Check sheet for the modelled part. Datum: model origin and axes. Units: mm. A direction names the side the tool comes from. Round coordinates to 2 decimals unless told otherwise and drop trailing zeros. Loops run counter-clockwise (first coordinate to the right, second up) from the corner with the lowest first, then second, coordinate; pieces in that order, holes last. Notation, with made-up numbers: (-36.75, -27.5) -> (7.25, -27.5) arc R22 cw to (7.25, -6.5) -> close; hole circle Ø8 at (85.25, 69). An arc over 180 degrees is marked (long way). One line per item, written item: value. Start each with the question number.
1. Cross-section at C-C on x = -41.5. Record the cut outline in (y, z).
2. Set-up check for faces 5 (the face through (-76, 2.845, 2)), 6 (the face through (76.353, 1.402, -1.021)): record each of +Z, -Z, +X, -X, +Y, -Y from which the full face is reachable in a straight line by a thin tool's end or side.
3. Cross-section at A-A on x = 0. Record the cut outline in (y, z).
4. Cross-section at B-B on z = 0. Record the cut outline in (x, y), then the cut area to 3 significant figures.
5. Material ranges on L1, parallel to X at y = 1.2, z = 0; L2, parallel to X at y = 4.2, z = 0; L3, parallel to Z at x = 51, y = 0.5, recorded low to high.
6. Go/stop test with flat-tipped pins: pin 1 (3.5 mm diameter, centred on x = -1.5, z = -75, fed in from +Y); pin 2 (11.5 mm diameter, centred on x = 74.75, z = 0, fed in from +Y); pin 3 (3 mm diameter, centred on y = 2.5, z = 62, fed in from -X); pin 4 (1 mm diameter, centred on y = 2, z = -14, fed in from -X). Record where each tip stops, or that it passes through.
7. Release check for a two-part mould opening along X. For faces 1 (the face through (32.42, 3.13, 62.33)), 2 (the face through (-1.368, 4.622, -71.452)), 3 (the face through (-6, 6.35, -71)), 4 (the face through (-10.317, 3.131, -78.574)) record: +X half, -X half, draft (parallel to the pull), parting line (faces both ways), or undercut.
8. Cross-section at D-D on z = 57. Record the cut outline in (x, y).
from build123d import *

# Parameters (mm, degrees)
SKETCH1_R                                      = 79.248
SKETCH1_R_2                                    = 70.2564
EXTRUDE2_DEPTH                                 = 6.35
CBORE_FOR_6_SOCKET_HEAD_CAP_SCREW1_D           = 3.7973
CBORE_FOR_6_SOCKET_HEAD_CAP_SCREW1_CBORE_D     = 7.14502
CBORE_FOR_6_SOCKET_HEAD_CAP_SCREW1_CBORE_DEPTH = 3.5052


with BuildPart() as part:
    # Sketch1 → Extrude2 (new body)
    with BuildSketch(Plane(origin=(0, 0, 0), x_dir=(1, 0, 0), z_dir=(0, 1, 0))):
        Circle(SKETCH1_R)
        Circle(SKETCH1_R_2, mode=Mode.SUBTRACT)
    extrude(amount=EXTRUDE2_DEPTH)

    # CBORE for #6 Socket Head Cap Screw1 (through all)
    with Locations(Plane(origin=(0, 6.35, -74.7522), x_dir=(0, 0, 1), z_dir=(0, 1, 0))):
        with Locations((0, 0), (149.5044, 0), (74.7522, 74.7522), (74.7522, -74.7522)):
            CounterBoreHole(CBORE_FOR_6_SOCKET_HEAD_CAP_SCREW1_D / 2, CBORE_FOR_6_SOCKET_HEAD_CAP_SCREW1_CBORE_D / 2, CBORE_FOR_6_SOCKET_HEAD_CAP_SCREW1_CBORE_DEPTH)


solid = part.part
Taken from the geometry:
1. outline: (0, -67.51) -> (6.35, -67.51) -> (6.35, -56.69) -> (0, -56.69) -> close; (0, 56.69) -> (6.35, 56.69) -> (6.35, 67.51) -> (0, 67.51) -> close
2. face 5: +Y
2. face 6: +Y, -Y
3. outline: (0, -79.25) -> (6.35, -79.25) -> (6.35, -78.32) -> (2.84, -78.32) -> (2.84, -76.65) -> (0, -76.65) -> close; (0, -72.85) -> (2.84, -72.85) -> (2.84, -71.18) -> (6.35, -71.18) -> (6.35, -70.26) -> (0, -70.26) -> close; (0, 70.26) -> (6.35, 70.26) -> (6.35, 71.18) -> (2.84, 71.18) -> (2.84, 72.85) -> (0, 72.85) -> close; (0, 76.65) -> (2.84, 76.65) -> (2.84, 78.32) -> (6.35, 78.32) -> (6.35, 79.25) -> (0, 79.25) -> close
4. outline: (-79.25, 0) -> (-76.65, 0) -> (-76.65, 2.84) -> (-78.32, 2.84) -> (-78.32, 6.35) -> (-79.25, 6.35) -> close; (-72.85, 0) -> (-70.26, 0) -> (-70.26, 6.35) -> (-71.18, 6.35) -> (-71.18, 2.84) -> (-72.85, 2.84) -> close; (70.26, 0) -> (72.85, 0) -> (72.85, 2.84) -> (71.18, 2.84) -> (71.18, 6.35) -> (70.26, 6.35) -> close; (76.65, 0) -> (79.25, 0) -> (79.25, 6.35) -> (78.32, 6.35) -> (78.32, 2.84) -> (76.65, 2.84) -> close
4. area: 42.5 mm2
5. L1: x = -79.25 to -76.65, -72.85 to -70.26, 70.26 to 72.85, 76.65 to 79.25
5. L2: x = -79.25 to -78.32, -71.18 to -70.26, 70.26 to 71.18, 78.32 to 79.25
5. L3: z = -60.66 to -48.32, 48.32 to 60.66
6. pin 1: stops at y = 2.84
6. pin 2: stops at y = 6.35
6. pin 3: stops at x = -51.19
6. pin 4: stops at x = -78.09
7. face 1: undercut
7. face 2: undercut
7. face 3: draft
7. face 4: parting line
8. outline: (-55.06, 0) -> (-41.07, 0) -> (-41.07, 6.35) -> (-55.06, 6.35) -> close; (41.07, 0) -> (55.06, 0) -> (55.06, 6.35) -> (41.07, 6.35) -> close
